Source: CAD feature listing. Evaluate the final solid. Frame: model axes, mm. A direction names the side the tool comes from. Give positions to 0.01 mm unless a question says otherwise; leave off trailing zeros. Order: outer loops, then holes, each group sorted by start corner. A loop starts at its lowest first (then second) coordinate and runs counter-clockwise, first axis right, second up. Notation, with made-up numbers: M 89,46 L 111,46 A9 cw 111,59 Z; hole C 1.25,34 d10. An arc over 180 degrees is marked long. Answer in a Markdown table with one row per item. Add a question column.
(1) Pin query (flat end, axial travel): P1, Ø10, axis at y = 112, z = 2, coming from the +X side; P2, Ø10, axis at x = -87, z = -60, coming from the +Y side; P3, Ø12.5, axis at x = -9, y = 201, coming from the -Z side. Return the tip coordinate at first contact, or that it passes through.
(2) Section query A-A, the plane x = -57.15. Return loops of the section in (y, z).
(3) Material intervals for line 1 along Y through (x, z) = (-57, 39); line 2 along Y through (x, z) = (-58, 3.5); line 3 along X through (y, z) = (89.5, -76), sorted ascending.
(4) Mould query, pull axis Y, two halves, no side actions, for faces 1 (the face through (-97.9, 57.4, 39.8)), 2 (the face through (-13, 200, 26.882)), 3 (the face through (46, 37.592, -50)). Classes: pulls with the +Y half, pulls with the -Y half, needs draft (parallel to the pull), parting line crosses it, or undercut.
(5) Section query D-D, the plane y = 136. Return loops of the section in (x, z), plus the area to 3 significant figures.
(6) Set-up query: faces 4 (the face through (-88.9, 200, 39)), 5 (the face through (-46, 124, 26.882)), 6 (the face through (-101, 200, 26.882)). Return all of +Z, -Z, +X, -X, +Y, -Y with unobstructed straight access to the full face (end or side cutting, diameter ignored); none if empty.
(7) Section query C-C, the plane y = 112.5. Return loops of the section in (x, z).
(8) Section query B-B, the plane z = -57. Return loops of the section in (x, y), plus the area to 3 significant figures.
from build123d import *

# Parameters (mm, degrees)
F0_W      = 76.2
F0_H      = 50.8
F0_R      = 12.7
F1_DEPTH  = 184.15
F2_R      = 51.343595
F2_R_2    = 35.929937
F3_DEPTH  = 25.4
F3_FACE_R = 35.929937
F4_DEPTH  = 311.15
F5_W      = 25.4
F5_H      = 25.4
F6_DEPTH  = 32.004
F7_W      = 76.2
F7_H      = 50.8
F7_R      = 12.7
F8_DEPTH  = 37.592
F9_DEPTH  = 0.762


with BuildPart() as f1:
    # F0 (on Front) → F1 (new body)
    with BuildSketch(Plane.XZ):
        Polygon((0, 52.28221), (-114.3, 52.28221), (-114.3, -87.41779), (0, -87.41779), (0, -36.61779), align=None)
        with Locations((38.1, -62.01779)):
            Rectangle(F0_W, F0_H)
        with Locations((38.1, -62.01779)):
            Circle(F0_R, mode=Mode.SUBTRACT)
    extrude(amount=-F1_DEPTH)

    # F2 (on face) → F3 (cut)
    with BuildSketch(Plane.XY.offset(52.28221)):
        with Locations((-57.15, 88.635586)):
            Circle(F2_R)
        with Locations((-57.15, 88.635586)):
            Circle(F2_R_2, mode=Mode.SUBTRACT)
    extrude(amount=-F3_DEPTH, mode=Mode.SUBTRACT)

    # F3_face (on face) → F4 (cut)
    with BuildSketch(Plane(origin=(-57.15, 88.635586, 52.28221), x_dir=(1, 0, 0), z_dir=(0, 0, 1))):
        Circle(F3_FACE_R)
    extrude(amount=-F4_DEPTH, mode=Mode.SUBTRACT)

    # F5 (on face) → F6 (join)
    with BuildSketch(Plane(origin=(0, 184.15, 0), x_dir=(-1, 0, 0), z_dir=(0, 1, 0))):
        with Locations((12.7, 39.58221)):
            Rectangle(F5_W, F5_H)
        with Locations((101.6, 39.58221)):
            Rectangle(F5_W, F5_H)
    extrude(amount=F6_DEPTH)

    # F7 (on face) → F8 (cut)
    with BuildSketch(Plane.XZ):
        with Locations((38.1, -62.01779)):
            Rectangle(F7_W, F7_H)
        with Locations((38.1, -62.01779)):
            Circle(F7_R, mode=Mode.SUBTRACT)
    extrude(amount=-F8_DEPTH, mode=Mode.SUBTRACT)

    # F6_face (on face) → F9 (join)
    with BuildSketch(Plane(origin=(-114.3, 95.38549, -15.817237), x_dir=(0, -1, 0), z_dir=(-1, 0, 0))):
        Polygon((95.38549, 68.099447), (-120.76851, 68.099447), (-120.76851, 42.699447), (-88.76451, 42.699447), (-88.76451, -71.600553), (95.38549, -71.600553), align=None)
    extrude(amount=-F9_DEPTH)


solid = f1.part
Values follow:
| question | item | result |
|---|---|---|
| 1 | P1 | stops at x = 0 |
| 1 | P2 | stops at y = 184.15 |
| 1 | P3 | stops at z = 26.88 |
| 2 | outline | M 0,-87.42 L 52.71,-87.42 L 52.71,26.88 L 37.29,26.88 L 37.29,52.28 L 0,52.28 Z; M 124.57,-87.42 L 184.15,-87.42 L 184.15,52.28 L 139.98,52.28 L 139.98,26.88 L 124.57,26.88 Z |
| 3 | line 1 | y = 0 to 37.29, 139.98 to 184.15 |
| 3 | line 2 | y = 0 to 52.72, 124.56 to 184.15 |
| 3 | line 3 | x = -114.3 to -93.07, -21.23 to 76.2 |
| 4 | face 1 | undercut |
| 4 | face 2 | needs draft |
| 4 | face 3 | pulls with the -Y half |
| 5 | outline | M -114.3,-87.42 L 76.2,-87.42 L 76.2,-36.62 L 0,-36.62 L 0,52.28 L -37.33,52.28 L -37.33,26.88 L -76.97,26.88 L -76.97,52.28 L -114.3,52.28 Z; hole C 38.1,-62.02 d25.4 |
| 5 | area | 18,300 mm² |
| 6 | face 4 | +Z, -Z, +Y |
| 6 | face 5 | +Z |
| 6 | face 6 | -Z, +X, -X, +Y |
| 7 | outline | M -114.3,-87.42 L -84.01,-87.42 L -84.01,26.88 L -102.61,26.88 L -102.61,52.28 L -114.3,52.28 Z; M -30.29,-87.42 L 76.2,-87.42 L 76.2,-36.62 L 0,-36.62 L 0,52.28 L -11.69,52.28 L -11.69,26.88 L -30.29,26.88 Z; hole C 38.1,-62.02 d25.4 |
| 8 | outline | M -114.3,0 L 0,0 L 0,37.59 L 26.43,37.59 L 26.43,184.15 L -114.3,184.15 Z; M 49.77,37.59 L 76.2,37.59 L 76.2,184.15 L 49.77,184.15 Z; hole C -57.15,88.64 d71.86 |
| 8 | area | 24,700 mm² |
